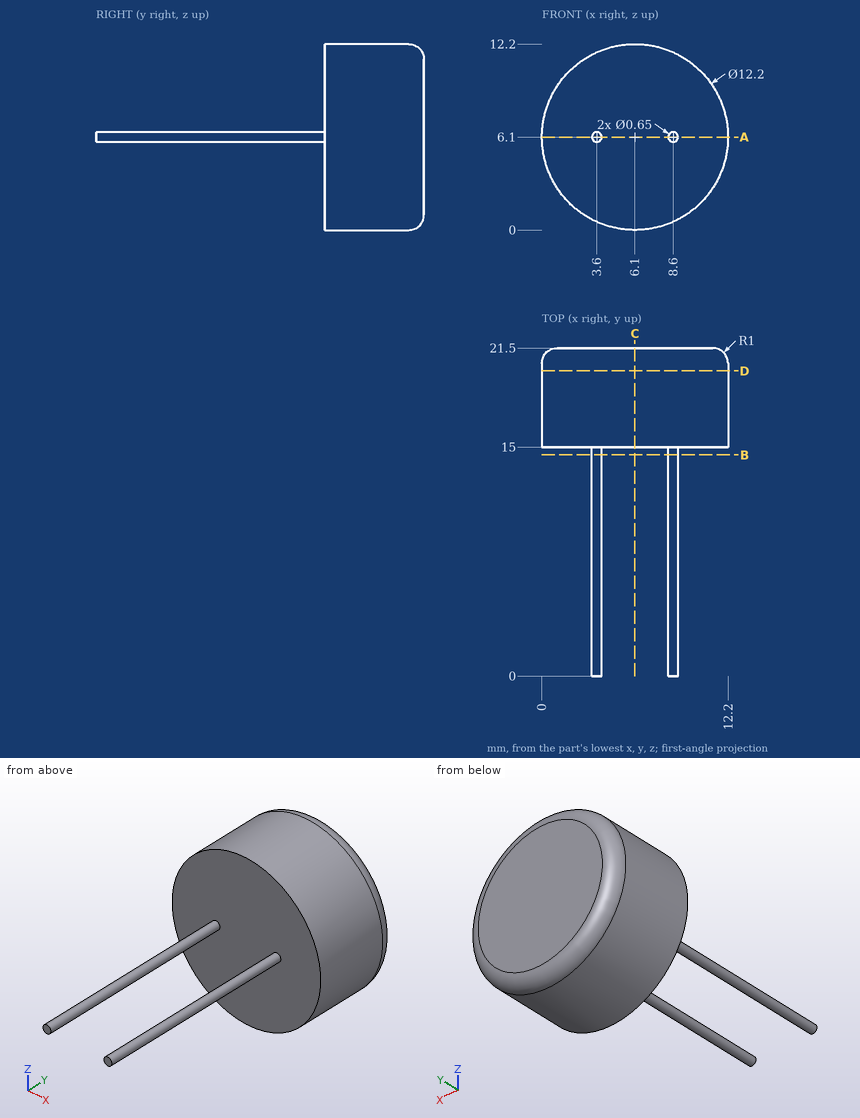
Here's the drawing with two shaded views (mm, measured from the low corner). I have some questions. Round coordinates to 2 decimals unless told otherwise and drop trailing zeros. Loops run counter-clockwise (first coordinate to the right, second up) from the corner with the lowest first, then second, coordinate; pieces in that order, holes last. Notation, with made-up numbers: M 10.25,-11 L 61.25,-11 A26 ccw 61.25,24 Z; hole C 53.25,56.25 d9. An arc over 180 degrees is marked long. Answer as a JSON object with one key per item and string values. Group by question number.
Q1. Imagine slicing it at B-B, the plane y = 14.5. Please give me the cut outline in (x, z) (3 decimals), then the cut area to 3 significant figures.
Q2. Imagine slicing it at D-D, the plane y = 20. Please give me the cut outline in (x, z).
Q3. Imagine slicing it at C-C, the plane x = 6.1. Please give me the cut outline in (y, z), then the cut area to 3 significant figures.
Q4. Please list where these lines run through material, in increasing order: L1, parallel to Y at x = 3.75, z = 5.25; L2, parallel to Z at x = 2.75, y = 17.25; L3, parallel to Z at x = 4.75, y = 16.5.
Q5. Will this pin go through, and if not, where does the flat tip stop? pin 1 (5 mm diameter, centred on y = 10.5, z = 3.5, fed in from -X).
Q6. Imagine slicing it at A-A, the plane z = 6.1. Please give me the cut outline in (x, y) (3 decimals), then the cut area to 3 significant figures.
Findings:
{
 "1": {"outline": "C 3.6,6.1 d0.65; C 8.6,6.1 d0.65", "area": "0.664 mm2"},
 "2": {"outline": "C 6.1,6.1 d12.2"},
 "3": {"outline": "M 15,0 L 20.5,0 A1 ccw 21.5,1 L 21.5,11.2 A1 ccw 20.5,12.2 L 15,12.2 Z", "area": "78.9 mm2"},
 "4": {"L1": "y = 15 to 21.5", "L2": "z = 1 to 11.2", "L3": "z = 0.15 to 12.05"},
 "5": {"pin 1": "stops at x = 3.29"},
 "6": {"outline": "M 0,15 L 3.275,15 L 3.275,0 L 3.925,0 L 3.925,15 L 8.275,15 L 8.275,0 L 8.925,0 L 8.925,15 L 12.2,15 L 12.2,20.5 A1 ccw 11.2,21.5 L 1,21.5 A1 ccw 0,20.5 Z", "area": "98.4 mm2"}
}
